The drawing under review shows one solid part. Ordinate dimensions are in mm from its lowest x, y, z. Coordinates: 2 decimals unless noted, no trailing zeros. Order: outer loops, then holes, each group sorted by start corner. A loop starts at its lowest first (then second) coordinate and runs counter-clockwise, first axis right, second up. Notation, with made-up numbers: (42, 50.5) -> (77, 50.5) arc R24 cw to (77, 71.5) -> close; hole circle Ø2 at (-25.75, 10.25). An arc over 180 degrees is marked (long way). Write item = value, one per line.
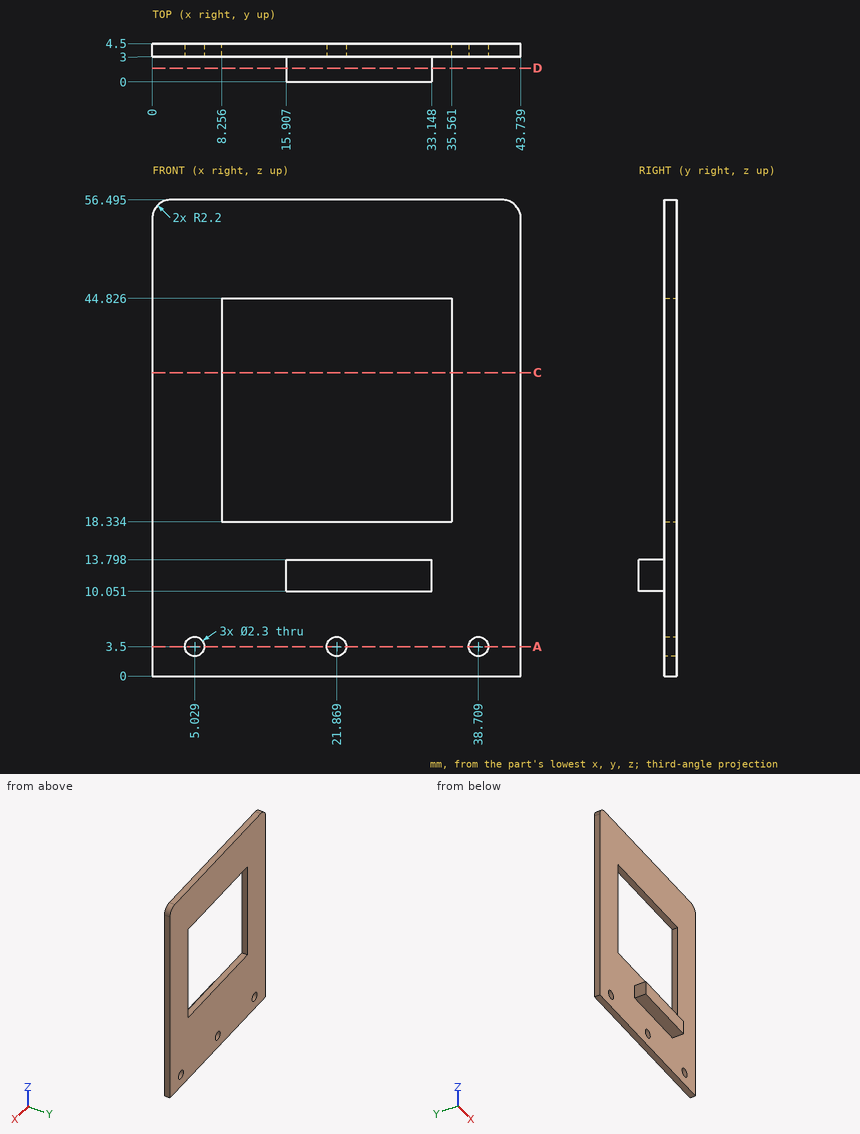
(1) We need section C-C (z = 36). Write out the cut boundary in (x, y) (1 decimal).
Report:
outline = (0, 3) -> (8.3, 3) -> (8.3, 4.5) -> (0, 4.5) -> close; (35.6, 3) -> (43.7, 3) -> (43.7, 4.5) -> (35.6, 4.5) -> close
(2) We need section D-D (y = 1.65). Write out the cut boundary in (x, z), and give its area (3 significant figures).
Report:
outline = (15.91, 10.05) -> (33.15, 10.05) -> (33.15, 13.8) -> (15.91, 13.8) -> close
area = 64.6 mm²
(3) For L1, parallel to X at y = 3.9, z = 3.5; L2, parallel to X at y = 3.2, z = 25.5 (1 decimal); L3, parallel to Z at x = 28, y = 4.3 (1 decimal), list the stretches that pass through material, from the lowest coordinate up.
Report:
L1 = 0 to 3.88, 6.18 to 20.72, 23.02 to 37.56, 39.86 to 43.74
L2 = 0 to 8.3, 35.6 to 43.7
L3 = 0 to 18.3, 44.8 to 56.5
(4) Insertion check: pin 1 (0.9 mm diameter, centred on y = 1, z = 11.5, fed in from -X); pin 2 (2 mm diameter, centred on x = 27, z = 19, fed in from -Y); pin 3 (2.5 mm diameter, centred on x = 27, y = 1.5, fed in from -Z). Each pin has a flat end and moves straight along its axis. Give the tip position at first contact, or say it passes through.
Report:
pin_1 = 15.91
pin_2 = 3
pin_3 = 10.05
(5) We need section A-A (z = 3.5). Write out the cut boundary in (x, y).
Report:
outline = (0, 3) -> (3.88, 3) -> (3.88, 4.5) -> (0, 4.5) -> close; (6.18, 3) -> (20.72, 3) -> (20.72, 4.5) -> (6.18, 4.5) -> close; (23.02, 3) -> (37.56, 3) -> (37.56, 4.5) -> (23.02, 4.5) -> close; (39.86, 3) -> (43.74, 3) -> (43.74, 4.5) -> (39.86, 4.5) -> close
